```python
from build123d import *

# Parameters (mm, degrees)
BOSS_EXTRUDE1_DEPTH     = 5
CUT_EXTRUDE1_DEPTH      = 164.77752047
CUT_EXTRUDE1_DEPTH_BACK = 164.77752047
SKETCH2_R               = 2
SKETCH2_R_2             = 5


with BuildPart() as part:
    # Sketch1 → Boss-Extrude1 (new, symmetric)
    with BuildSketch(Plane.XY):
        with BuildLine():
            Line((5.466587816, 13.968407842), (-40.567976281, 31.984203921))
            ThreePointArc((-40.567976281, 31.984203921), (-49.796460718, 28.75), (-47.983121256, 19.140796079))
            Line((-47.983121256, 19.140796079), (-9.363702133, -11.718407842))
            ThreePointArc((-9.363702133, -11.718407842), (-8.248107249, -12.528716088), (-7.062819473, -13.233162173))
            Line((-7.062819473, -13.233162173), (125.195264252, -83.822108115))
            ThreePointArc((125.195264252, -83.822108115), (138.564064606, -80), (135.189707152, -66.511225218))
            Line((135.189707152, -66.511225218), (7.928844877, 12.733162173))
            ThreePointArc((7.928844877, 12.733162173), (6.726132784, 13.407428455), (5.466587816, 13.968407842))
        make_face()
    extrude(amount=BOSS_EXTRUDE1_DEPTH, both=True)

    # Sketch2 → Cut-Extrude1 (cut, two sides: drawn at the far end of the back side and taken through both)
    with BuildSketch(Plane.XY.offset(-CUT_EXTRUDE1_DEPTH_BACK)):
        with Locations((-43.301270189, 25)):
            Circle(SKETCH2_R)
        Circle(SKETCH2_R_2)
    extrude(amount=CUT_EXTRUDE1_DEPTH + CUT_EXTRUDE1_DEPTH_BACK, mode=Mode.SUBTRACT)


solid = part.part
```
The listing builds one solid part. Answer for the finished solid, in the listing's coordinates (mm). Give positions to 0.01 mm unless a question says otherwise; leave off trailing zeros. Write each loop counter-clockwise with the first axis right and the second up, starting at its lowest first coordinate (ties: lowest second). Pieces come first, ordered by that corner, then holes. Notation, with made-up numbers: (-16, 11.5) -> (40, 11.5) arc R11 cw to (40, 25.5) -> close; hole circle Ø10 at (-7, 36.25). An arc over 180 degrees is marked (long way). Write item = value, one per line. Start each with the question number.
1) Straight lines are drawn through the part: line 1 along Y through (x, z) = (3, -3); line 2 along Y through (x, z) = (-1, 4.25); line 3 along X through (y, z) = (4, 3). For each, find the intervals that lie inside material, in ascending order.
2) Each of these flat-tipped pins is pushed along its axis until it touches: pin 1 (4 mm diameter, centred on y = -32, z = -2.5, fed in from +X); pin 2 (2 mm diameter, centred on x = 80, z = 0, fed in from -Y); pin 3 (2 mm diameter, centred on x = 77, z = -2, fed in from -Y). Where does it stop, or does it pass through?
3) The part is cut by section C-C, the plane x = 0. Determine the outline of the cut face in (y, z).
4) The part is cut by section B-B, the plane y = 25. Determine the outline of the cut face in (x, z), and give its area (3 significant figures).
5) The part is cut by section D-D, the plane y = -25. Determine the outline of the cut face in (x, z), and give its area (3 significant figures).
6) The part is cut by section A-A, the plane z = -3.25. Determine the outline of the cut face in (x, y).
7) Determine the mould class of faces 1 (the face through (72.45, -27.444, 0.07)), 2 (the face through (-41.454, 24.234, -0.07)), 3 (the face through (138.45, -80.19, 0.07)) for opening direction X: +X half, -X half, draft (parallel to the pull), parting line (faces both ways), or undercut.
Solutions:
q1.line_1 = -18.6 to -4, 4 to 14.93
q1.line_2 = -16.47 to -4.9, 4.9 to 16.5
q1.line_3 = -29.03 to -3, 3 to 21.95
q2.pin_1 = 82.98
q2.pin_2 = -60.23
q2.pin_3 = -58.63
q3.outline = (-17, -5) -> (-5, -5) -> (-5, 5) -> (-17, 5) -> close; (5, -5) -> (16.11, -5) -> (16.11, 5) -> (5, 5) -> close
q4.outline = (-50.8, -5) -> (-45.3, -5) -> (-45.3, 5) -> (-50.8, 5) -> close; (-41.3, -5) -> (-22.72, -5) -> (-22.72, 5) -> (-41.3, 5) -> close
q4.area = 241 mm²
q5.outline = (14.98, -5) -> (68.53, -5) -> (68.53, 5) -> (14.98, 5) -> close
q5.area = 535 mm²
q6.outline = (-47.98, 19.14) -> (-9.36, -11.72) arc R15 ccw to (-7.06, -13.23) -> (125.2, -83.82) arc R10 ccw to (135.19, -66.51) -> (7.93, 12.73) arc R15 ccw to (5.47, 13.97) -> (-40.57, 31.98) arc R7.5 ccw to start; hole circle Ø4 at (-43.3, 25); hole circle Ø10 at (0, 0)
q7.face_1 = +X half
q7.face_2 = undercut
q7.face_3 = parting line
